Source: CAD feature listing. Evaluate the final solid. Frame: model axes, mm. A direction names the side the tool comes from. Give positions to 0.01 mm unless a question says otherwise; leave off trailing zeros. Write each loop counter-clockwise with the first axis right and the second up, starting at its lowest first coordinate (ties: lowest second). Pieces come first, ordered by that corner, then holes. Notation, with made-up numbers: (23.5, 12.25) -> (53.5, 12.25) arc R6 ccw to (53.5, 18.25) -> close; hole circle Ø10 at (-27, -8). An arc over 180 degrees is marked (long way). Answer as a JSON object with one key per item and string values. Group by question number.
Item 1: Ray query, probe 1 along Y at (x, z) = (28.5, -5) (1 decimal); probe 2 along Z at (x, y) = (-6, -11.75); probe 3 along X at (y, z) = (-14.5, 11). Return the intervals inside material, ascending. Write a range as from..to.
Item 2: Access query for faces 1 (the face through (0, -28.575, 0)), 2 (the face through (0, -17, 12)), 3 (the face through (12.7, -23, -10)). Directions: +Z, -Z, +X, -X, +Y, -Y. A direction counts if a zero-diameter tool reaches every point of the face in a straight line with its end or side. Return the directions, or none.
Item 3: Section query C-C on y = -9.5. Return the cut outline in (x, z), plus the area to 3 significant figures.
Item 4: Pull-direction query (Z, two-part tool) for faces 4 (the face through (0.462, -1.449, 17.522)), 5 (the face through (-36.65, -27.05, 0.2)), 6 (the face through (26, -19, -13.97)); classes: pulls with the +Z half, pulls with the -Z half, needs draft (parallel to the pull), parting line crosses it, or undercut.
Item 5: First-contact query: pin 1 Ø10 at (x, y) = (8.5, -4) entering from -Z; pin 2 Ø3 at (x, z) = (-21.5, -0.5) entering from +Y (3 decimals). Flat tips, straight axial feed; report the tip coordinate or a pass-through.
Item 6: Section query D-D on z = 5.5. Return the cut outline in (x, y) (3 decimals), plus the area to 3 significant figures.
Item 7: Section query B-B on z = -1. Return the cut outline in (x, y) (1 decimal).
from build123d import *

# Parameters (mm, degrees)
F0_W      = 76.2
F0_H      = 38.1
F0_W_2    = 53.34
F0_H_2    = 19.304
F1_DEPTH  = 12.7
F2_W      = 76.2
F2_H      = 38.1
F3_DEPTH  = 12.7
F4_W      = 53.34
F4_H      = 3.175
F5_DEPTH  = 31.05
F5_FACE_W = 76.2
F5_FACE_H = 3.175
F6_DEPTH  = 7.05
F7_R      = 5.08
F8_W      = 9.2075
F8_H      = 13.97
F9_DEPTH  = 25.4


with BuildPart() as f1:
    # F0 (on Front) → F1 (new body)
    with BuildSketch(Plane.XZ):
        Rectangle(F0_W, F0_H)
        Rectangle(F0_W_2, F0_H_2, mode=Mode.SUBTRACT)
    extrude(amount=F1_DEPTH)

    # F2 (on face) → F3 (join)
    with BuildSketch(Plane.XZ.offset(12.7)):
        Rectangle(F2_W, F2_H)
        Polygon((-26.67, 12), (26.67, 12), (26.67, 9.652), (26.67, -9.652), (26.67, -12), (-26.67, -12), (-26.67, -9.652), (-26.67, 9.652), align=None, mode=Mode.SUBTRACT)
    extrude(amount=F3_DEPTH)

    # F4 (on face) → F5 (join, through all)
    with BuildSketch(Plane(origin=(0, 0, 12), x_dir=(1, 0, 0), z_dir=(0, 0, -1))):
        Polygon((38.1, 22.225), (38.1, 28.575), (-38.1, 28.575), (-38.1, 22.225), (-26.67, 22.225), (-26.67, 25.4), (26.67, 25.4), (26.67, 22.225), align=None)
        with Locations((0, 23.8125)):
            Rectangle(F4_W, F4_H)
    extrude(amount=F5_DEPTH)

    # F5_face (on face) → F6 (join, through all)
    with BuildSketch(Plane(origin=(0, -26.9875, 12), x_dir=(1, 0, 0), z_dir=(0, 0, 1))):
        Rectangle(F5_FACE_W, F5_FACE_H)
    extrude(amount=F6_DEPTH)

    # F7
    f7_edges = [f1.edges().sort_by_distance(p)[0] for p in [
        (0, 0, 19.05),
        (38.1, -14.2875, 19.05),
        (0, -28.575, 19.05),
        (-38.1, -14.2875, 19.05),
        (-38.1, 0, 0),
        (38.1, 0, 0),
        (0, 0, -19.05),
        (38.1, -14.2875, -19.05),
        (-38.1, -14.2875, -19.05),
        (0, -28.575, -19.05),
        (38.1, -28.575, 0),
        (-38.1, -28.575, 0),
    ]]
    fillet(f7_edges, radius=F7_R)

    # F8 (on face) → F9 (cut)
    with BuildSketch(Plane.YZ.offset(38.1)):
        with Locations((-18.89125, -6.985)):
            Rectangle(F8_W, F8_H)
    extrude(amount=-F9_DEPTH, mode=Mode.SUBTRACT)


solid = f1.part
Worked answers:
{
 "1": {"probe 1": "-28.6..-23.5, -14.3..0", "probe 2": "-19.05..-9.65, 9.65..19.05", "probe 3": "-38.1..-26.67, 26.67..38.1"},
 "2": {"face 1": "+Z, -Z, +X, -X, -Y", "face 2": "none", "face 3": "+X"},
 "3": {"outline": "(-38.1, -13.97) arc R5.08 ccw to (-33.02, -19.05) -> (33.02, -19.05) arc R5.08 ccw to (38.1, -13.97) -> (38.1, 13.97) arc R5.08 ccw to (33.02, 19.05) -> (-33.02, 19.05) arc R5.08 ccw to (-38.1, 13.97) -> close; hole (-26.67, -9.65) -> (26.67, -9.65) -> (26.67, 9.65) -> (-26.67, 9.65) -> close", "area": "1,850 mm^2"},
 "4": {"face 4": "pulls with the +Z half", "face 5": "needs draft", "face 6": "undercut"},
 "5": {"pin 1": "z = -19.05", "pin 2": "y = -22.225"},
 "6": {"outline": "(-38.1, -23.495) arc R5.08 ccw to (-33.02, -28.575) -> (33.02, -28.575) arc R5.08 ccw to (38.1, -23.495) -> (38.1, -5.08) arc R5.08 ccw to (33.02, 0) -> (26.67, 0) -> (26.67, -22.225) -> (-26.67, -22.225) -> (-26.67, 0) -> (-33.02, 0) arc R5.08 ccw to (-38.1, -5.08) -> close", "area": "970 mm^2"},
 "7": {"outline": "(-38.1, -23.5) arc R5.1 ccw to (-33, -28.6) -> (33, -28.6) arc R5.1 ccw to (38.1, -23.5) -> (12.7, -23.5) -> (12.7, -22.2) -> (-26.7, -22.2) -> (-26.7, 0) -> (-33, 0) arc R5.1 ccw to (-38.1, -5.1) -> close; (26.7, -14.3) -> (38.1, -14.3) -> (38.1, -5.1) arc R5.1 ccw to (33, 0) -> (26.7, 0) -> close"}
}
